Autodesk Inventor part; units mm, degrees
ref_plane "YZ Plane" through (0, 0, 0) normal (1, 0, 0) x (0, 1, 0)
ref_plane "XZ Plane" through (0, 0, 0) normal (0, 1, 0) x (-1, 0, 0)
ref_plane "XY Plane" through (0, 0, 0) normal (0, 0, 1) x (1, 0, 0)
sketch "Sketch2" plane through (0, 0, 0) normal (0, 0, 1) x (1, 0, 0)
  circle A0 centre (-58.827, 33.0516) radius 2.1971
  circle A1 centre (-20.727, 33.0516) radius 2.0955
  circle A2 centre (62.1938, 43.4026) radius 2.1844
  circle A3 centre (52.9267, 52.0864) radius 2.1844
  circle A4 centre (18.7744, -2.9332) radius 2.1844
  circle A5 centre (9.5073, 5.7507) radius 2.1844
  circle A6 centre (-90.577, 26.7016) radius 2.0955
  circle A7 centre (-1.677, 39.4016) radius 2.0955
  arc A8 (-91.6831, 32.9546) -> (-92.238, 20.5727) centre (-90.577, 26.7016) ccw
  arc A9 (57.2686, 56.72) -> (51.8206, 58.3394) centre (52.9267, 52.0864) ccw
  arc A10 (66.8274, 39.0606) -> (66.5358, 48.0361) centre (62.1938, 43.4026) ccw
  arc A11 (17.1134, -9.0622) -> (23.408, -7.2752) centre (18.7744, -2.9332) ccw
  line L0 (-92.238, 20.5727) -> (17.1134, -9.0622)
  line L1 (66.8274, 39.0606) -> (23.408, -7.2752)
  line L2 (66.5358, 48.0361) -> (57.2686, 56.72)
  line L3 (51.8206, 58.3394) -> (-91.6831, 32.9546)
  dimension "d17" = 4.191
  dimension "d18" = 4.191
  dimension "d19" = 12.7
  dimension "d20" = 12.7
  dimension "d21" = 12.7
  dimension "d22" = 12.7
extrude "Extrusion2" add sketch "Sketch2" along normal blind 1.5875
properties part number "1-Gearbox"
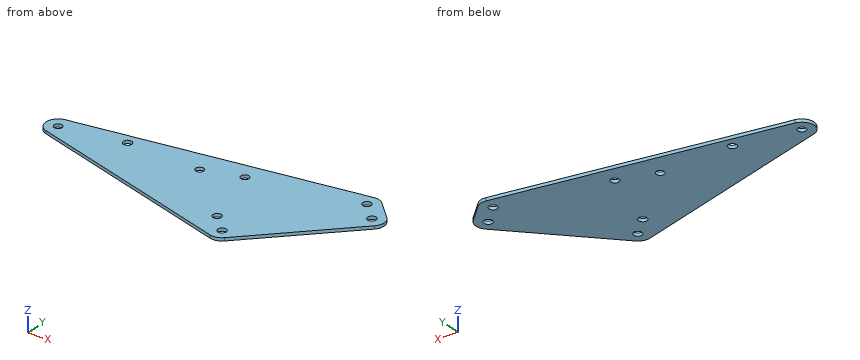
Verification items for the finished model (mm, model axes). Give positions to 0.01 mm unless a question says otherwise; leave off trailing zeros. Write each loop counter-clockwise with the first axis right and the second up, starting at its lowest first coordinate (ties: lowest second). Pieces come first, ordered by that corner, then holes. Notation, with made-up numbers: (2.5, 18) - (57.5, 18) arc R21 cw to (57.5, 43) - close; hole circle Ø5 at (17, 80). An arc over 180 degrees is marked (long way). Put each result on its own line as item: value.
Q1. Scan lines: probe 1 along Y at (x, z) = (-23, 0.75); probe 2 along Y at (x, z) = (2.5, 1.25); probe 3 along X at (y, z) = (30, 1). Record each from-to range of solid material in increasing order. Write a range as from..to.
Result:
probe 1: 1.81..45.1
probe 2: -5.1..49.61
probe 3: -96..58.34
Q2. Section check A-A on x = -2. Record the cut outline in (y, z).
Result:
outline: (-3.88, 0) - (37.33, 0) - (37.33, 1.59) - (-3.88, 1.59) - close; (41.47, 0) - (48.82, 0) - (48.82, 1.59) - (41.47, 1.59) - close
Q3. Section check B-B on z = 0.8. Count the separate pieces of the cut face and the enclosed holes in it, and give its area (3 significant figures).
Result:
separate pieces: 1
enclosed holes: 8
area: 6,060 mm2
Q4. Depth check by flat-ended pin: P1, Ø2.5, axis at x = -1.68, y = 39.4, coming from the +Z side. Enter the tip coordinate at first touch or a pass-through.
Result:
P1: through
Q5. Section check C-C on x = -24.5. Record the cut outline in (y, z), and give its area (3 significant figures).
Result:
outline: (2.22, 0) - (44.84, 0) - (44.84, 1.59) - (2.22, 1.59) - close
area: 67.7 mm2
Q6. Section check D-D on x = 44. Record the cut outline in (y, z).
Result:
outline: (14.7, 0) - (56.96, 0) - (56.96, 1.59) - (14.7, 1.59) - close
